The model under review builds one solid part; all positions refer to its coordinate system, in mm. A direction names the side the tool comes from. Round coordinates to 2 decimals unless told otherwise and drop trailing zeros. Order: outer loops, then holes, each group sorted by start corner. A loop starts at its lowest first (then second) coordinate and runs counter-clockwise, first axis right, second up.
1) Consider section A-A (z = 0.03). Give the boundary of the cut face in (x, y), then the cut area to 3 significant figures.
2) Consider section C-C (y = 13.5). Give the number of separate pieces and of enclosed holes in the cut face, then the cut area to 3 significant figures.
3) Consider section B-B (x = -2.5). Give the boundary of the cut face in (y, z) (3 decimals).
4) Consider section D-D (z = -7.5). Give the boundary of the cut face in (x, y), then the cut area to 3 significant figures.
5) To check wall thickness, follow L1, parallel to X at y = 9.25, z = 19; L2, parallel to Z at x = -9.5, y = 3.75; L3, parallel to Z at x = 5, y = 10.25. State the ranges of each line that lie inside material, in increasing order.
6) Machinability: for faces 1 (the face through (-4, 7, -27.45)), 2 (the face through (-8.32, 7.93, -28.5)), 3 (the face through (15, 10, -24)), 4 (the face through (6.68, 7.93, 28.5)), 5 (the face through (-15, 5.4, 0)), which of the approach directions +Z, -Z, +X, -X, +Y, -Y give a long, thin tool a straight path to every point of the face, cutting with its end or side? Answer none if there is none.
7) Mouldability with a two-part tool opening along X and no side actions: class faces 6 (the face through (-14.57, 12.64, 28.24)), 7 (the face through (-8, 7.95, -27.98)), 8 (the face through (-15, 10, -24)) as pulls with the +X half, pulls with the -X half, needs draft (parallel to the pull), parting line crosses it, or undercut.
8) Clearance check with flat-ended pins moving along their axes: P1, Ø4, axis at y = 11.5, z = 18, coming from the +X side; P2, Ø0.6, axis at x = 0, y = 5, coming from the +Z side; P3, Ø0.6, axis at x = 0, z = 26, coming from the +Y side; P4, Ø4, axis at x = -5.5, z = 10, coming from the -Y side. State where each tip first meets the part, or that it passes through.
from build123d import *

# Parameters (mm, degrees)
SKETCH1_R           = 1.075
BOSS_EXTRUDE1_DEPTH = 29
CUT_EXTRUDE7_START  = -1.55
CUT_EXTRUDE7_DEPTH  = 54.9
BOSS_EXTRUDE2_DEPTH = 0.55
CUT_EXTRUDE8_REACH  = 47.442
SKETCH4_W           = 3.45
SKETCH4_H           = 15
SKETCH4_W_2         = 18.25
SKETCH4_H_2         = 16
SKETCH5_R           = 3.95
CUT_EXTRUDE9_DEPTH  = 0.5
SKETCH6_R           = 1.65
CUT_EXTRUDE10_DEPTH = 36.632283115
SKETCH10_W          = 2
SKETCH10_H          = 7.4
CUT_EXTRUDE11_DEPTH = 1.55
SKETCH12_R          = 1.075
CUT_EXTRUDE12_DEPTH = 1.55
SKETCH14_W          = 7.23
SKETCH14_H          = 2.9
CUT_EXTRUDE13_DEPTH = 1


with BuildPart() as part:
    # Sketch1 → Boss-Extrude1 (new, symmetric)
    with BuildSketch(Plane.XY):
        with BuildLine():
            Line((-11, 14.14), (11, 14.14))
            ThreePointArc((11, 14.14), (14.535533906, 12.675533906), (16, 9.14))
            Line((16, 9.14), (16, 0))
            Line((16, 0), (-16, 0))
            Line((-16, 0), (-16, 9.14))
            ThreePointArc((-16, 9.14), (-14.535533906, 12.675533906), (-11, 14.14))
        make_face()
        with Locations(Location((-7.5, 7, 0), (0, 0, 180))):
            Circle(SKETCH1_R, mode=Mode.SUBTRACT)
        with Locations(Location((7.5, 7, 0), (0, 0, 180))):
            Circle(SKETCH1_R, mode=Mode.SUBTRACT)
    extrude(amount=BOSS_EXTRUDE1_DEPTH, both=True)

    # Sketch2 → Cut-Extrude7 (cut)
    with BuildSketch(Plane.XY.offset(29).offset(CUT_EXTRUDE7_START)):
        with BuildLine():
            Line((-14.7, 1), (14.7, 1))
            Line((14.7, 1), (14.7, 9.55))
            ThreePointArc((14.7, 9.55), (13.235533906, 13.085533906), (9.7, 14.55))
            Line((9.7, 14.55), (-9.7, 14.55))
            ThreePointArc((-9.7, 14.55), (-13.235533906, 13.085533906), (-14.7, 9.55))
            Line((-14.7, 9.55), (-14.7, 1))
        make_face()
    extrude(amount=-CUT_EXTRUDE7_DEPTH, mode=Mode.SUBTRACT)

    # Sketch3 → Boss-Extrude2 (add, symmetric)
    with BuildSketch(Plane(origin=(0, 0, 0), x_dir=(0, 0, -1), z_dir=(1, 0, 0))):
        Polygon((27.45, 14.068958196), (22.45, 14.068958196), (10, 5.068958196), (-10, 5.068958196), (-22.45, 14.068958196), (-27.45, 14.068958196), (-27.45, 1), (27.45, 1), align=None)
    extrude(amount=BOSS_EXTRUDE2_DEPTH, both=True)

    # Sketch4 → Cut-Extrude8 (cut, up to next)
    with BuildSketch(Plane(origin=(16, 0, 0), x_dir=(0, 0, -1), z_dir=(1, 0, 0)), mode=Mode.PRIVATE) as cut_extrude8_sk1:
        with Locations((-25.725, 13.9)):
            Rectangle(SKETCH4_W, SKETCH4_H)
    cut_extrude8_tool1 = extrude(cut_extrude8_sk1.sketch, amount=-CUT_EXTRUDE8_REACH, mode=Mode.PRIVATE) & part.part
    # Sketch4 → Cut-Extrude8 (cut, up to next)
    with BuildSketch(Plane(origin=(16, 0, 0), x_dir=(0, 0, -1), z_dir=(1, 0, 0)), mode=Mode.PRIVATE) as cut_extrude8_sk2:
        with Locations((0, 13.4)):
            Rectangle(SKETCH4_W_2, SKETCH4_H_2)
    cut_extrude8_tool2 = extrude(cut_extrude8_sk2.sketch, amount=-CUT_EXTRUDE8_REACH, mode=Mode.PRIVATE) & part.part
    # Sketch4 → Cut-Extrude8 (cut, up to next)
    with BuildSketch(Plane(origin=(16, 0, 0), x_dir=(0, 0, -1), z_dir=(1, 0, 0)), mode=Mode.PRIVATE) as cut_extrude8_sk3:
        with Locations((25.725, 13.9)):
            Rectangle(SKETCH4_W, SKETCH4_H)
    cut_extrude8_tool3 = extrude(cut_extrude8_sk3.sketch, amount=-CUT_EXTRUDE8_REACH, mode=Mode.PRIVATE) & part.part
    cut_extrude8_1 = cut_extrude8_tool1.solids().sort_by_distance((16, 13.9, 25.725))[0]
    add(cut_extrude8_1, mode=Mode.SUBTRACT)
    cut_extrude8_2 = cut_extrude8_tool2.solids().sort_by_distance((16, 13.4, 0))[0]
    add(cut_extrude8_2, mode=Mode.SUBTRACT)
    cut_extrude8_3 = cut_extrude8_tool3.solids().sort_by_distance((16, 13.9, -25.725))[0]
    add(cut_extrude8_3, mode=Mode.SUBTRACT)
    cut_extrude8 = cut_extrude8_1 + cut_extrude8_2 + cut_extrude8_3  # Cut-Extrude8 as one shape, for the pattern or mirror that repeats it

    # Mirror1: Cut-Extrude8 across plane
    add(cut_extrude8.mirror(Plane(origin=(0, 0, 0), x_dir=(0, 0, 1), z_dir=(1, 0, 0))), mode=Mode.SUBTRACT)

    # Sketch5 → Cut-Extrude9 (cut)
    with BuildSketch(Plane(origin=(0, 0, -29), x_dir=(-1, 0, 0), z_dir=(0, 0, -1))):
        with Locations((-7.5, 7)):
            Circle(SKETCH5_R)
        with Locations((7.5, 7)):
            Circle(SKETCH5_R)
    cut_extrude9 = extrude(amount=-CUT_EXTRUDE9_DEPTH, mode=Mode.SUBTRACT)

    # Mirror2: Cut-Extrude9 across plane
    add(cut_extrude9.mirror(Plane.XY), mode=Mode.SUBTRACT)

    # Sketch6 → Cut-Extrude10 (cut, through all)
    with BuildSketch(Plane(origin=(0, 1, 0), x_dir=(1, 0, 0), z_dir=(0, 1, 0))):
        with Locations(Location((-9, -0.03, 0), (0, 0, 270))):
            Circle(SKETCH6_R)
        with Locations(Location((9, -0.03, 0), (0, 0, 90))):
            Circle(SKETCH6_R)
    extrude(amount=-CUT_EXTRUDE10_DEPTH, mode=Mode.SUBTRACT)

    # Sketch10 → Cut-Extrude11 (cut)
    with BuildSketch(Plane.XY.offset(29)):
        with Locations((0, 4.7)):
            Rectangle(SKETCH10_W, SKETCH10_H)
    extrude(amount=-CUT_EXTRUDE11_DEPTH, mode=Mode.SUBTRACT)

    # Sketch12 → Cut-Extrude12 (cut)
    with BuildSketch(Plane(origin=(0, 0, -29), x_dir=(-1, 0, 0), z_dir=(0, 0, -1))):
        with Locations((-2.5, 2.5)):
            Circle(SKETCH12_R)
        with Locations((2.5, 2.5)):
            Circle(SKETCH12_R)
    extrude(amount=-CUT_EXTRUDE12_DEPTH, mode=Mode.SUBTRACT)

    # Sketch14 → Cut-Extrude13 (cut)
    with BuildSketch(Plane.XZ):
        with Locations((-7.635, 26)):
            Rectangle(SKETCH14_W, SKETCH14_H)
        with Locations((7.595, 26)):
            Rectangle(SKETCH14_W, SKETCH14_H)
    cut_extrude13 = extrude(amount=-CUT_EXTRUDE13_DEPTH, mode=Mode.SUBTRACT)

    # Mirror3: Cut-Extrude13 across plane
    add(cut_extrude13.mirror(Plane.XY), mode=Mode.SUBTRACT)


solid = part.part
Answer below:
1. outline: (-16, 0) - (-10.65, 0) - (-10.65, 1) - (-14.7, 1) - (-14.7, 5.4) - (-16, 5.4) - close; (-7.35, 0) - (7.35, 0) - (7.35, 1) - (0.55, 1) - (0.55, 5.07) - (-0.55, 5.07) - (-0.55, 1) - (-7.35, 1) - close; (10.65, 0) - (16, 0) - (16, 5.4) - (14.7, 5.4) - (14.7, 1) - (10.65, 1) - close
1. area: 41.3 mm2
2. separate pieces: 6
2. enclosed holes: 0
2. area: 137 mm2
3. outline: (0, -29) - (1.425, -29) - (1.425, -27.45) - (1, -27.45) - (1, 27.45) - (14.14, 27.45) - (14.14, 29) - (0, 29) - close; (3.575, -29) - (14.14, -29) - (14.14, -27.45) - (3.575, -27.45) - close
4. outline: (-16, 0) - (16, 0) - (16, 5.4) - (14.7, 5.4) - (14.7, 1) - (0.55, 1) - (0.55, 5.07) - (-0.55, 5.07) - (-0.55, 1) - (-14.7, 1) - (-14.7, 5.4) - (-16, 5.4) - close
4. area: 47.9 mm2
5. L1: x = -16 to -14.7, -0.55 to 0.55, 14.7 to 16
5. L2: z = -28.5 to -27.45, 27.45 to 28.5
5. L3: z = -29 to -27.45, 27.45 to 29
6. face 1: +Y
6. face 2: -Z
6. face 3: +X, +Y
6. face 4: +Z
6. face 5: +X, -X, +Y
7. face 6: pulls with the -X half
7. face 7: undercut
7. face 8: needs draft
8. P1: stops at x = 15.99
8. P2: stops at z = 27.45
8. P3: stops at y = 14.07
8. P4: stops at y = 0
